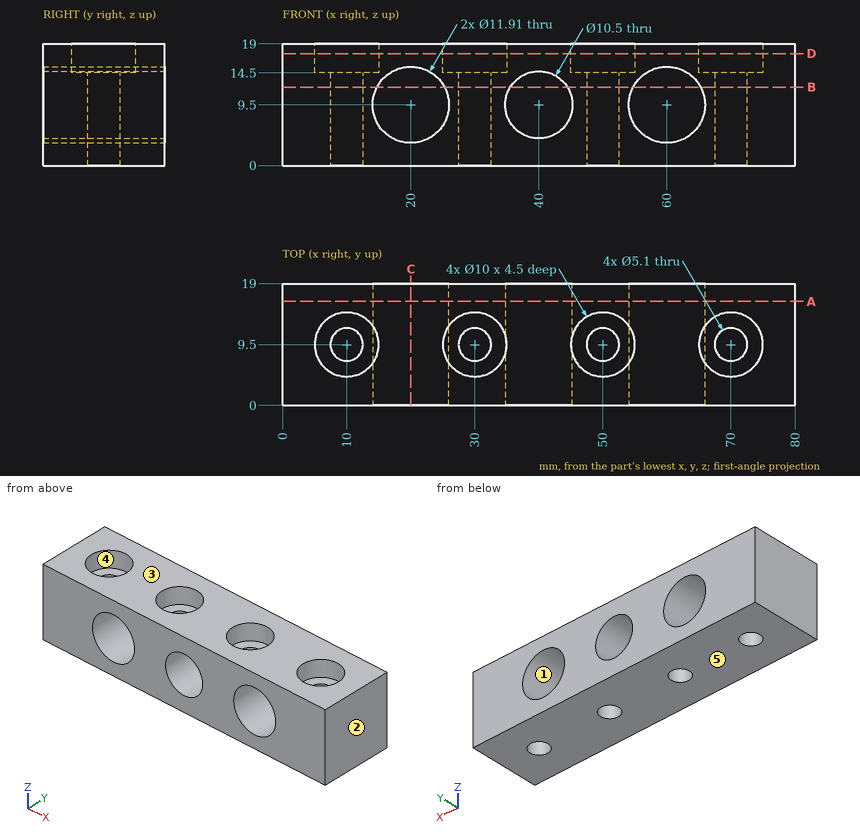
Answer from the drawing. Dimensions are ordinates in mm from the lowest x, y and z of the part. A direction names the side the tool comes from. Give positions to 0.01 mm unless a question says otherwise; leave off trailing zeros. Write each loop counter-clockwise with the first axis right and the second up, starting at its lowest first coordinate (ties: lowest second). Pieces come first, ordered by that corner, then holes. Notation, with made-up numbers: (-24, -15.5) - (9, -15.5) arc R20 ccw to (9, -8.5) - close; hole circle Ø8 at (-14, -36.5). An arc over 180 degrees is marked (long way). One line per item, written item: value. Start each with the question number.
1. Find section A-A (y = 16.25). Write down the section's boundary in (x, z) (3 decimals).
2. For the marked faces 4 and 5, determine the directions among +Z, -Z, +X, -X, +Y, -Y from which every point of the face is accessible in a straight line to the end or side of a thin tool.
3. For a pull along Z with two mould halves and no side action, classify the marked faces 1, 2 and 3 as +Z half, -Z half, draft (parallel to the pull), parting line (faces both ways), or undercut.
4. Find section B-B (z = 12.25). Write down the section's boundary in (x, y), then the cut area to 3 significant figures.
5. Consider probe 1 along X at (y, z) = (17.75, 9.75); probe 2 along Z at (x, y) = (60, 4) (3 decimals); probe 3 along X at (y, z) = (15.75, 6.5). Determine where each line is inside the solid, lowest interval first.
6. Find section C-C (x = 20). Write down the section's boundary in (y, z) (3 decimals), then the cut area to 3 significant figures.
7. Given pin 1 (8 mm diameter, centred on x = 30, y = 9.5, fed in from +Z); pin 2 (7 mm diameter, centred on x = 20, z = 9.5, fed in from +Y), each flat-ended and moving along its own axis, determine where each tip first touches the part or whether it passes through.
8. Find section D-D (z = 17.5). Write down the section's boundary in (x, y).
Geometry results:
1. outline: (0, 0) - (80, 0) - (80, 19) - (0, 19) - close; hole circle Ø11.91 at (20, 9.5); hole circle Ø10.5 at (40, 9.5); hole circle Ø11.91 at (60, 9.5)
2. face 4: +Z
2. face 5: -Z, +X, -X, +Y, -Y
3. face 1: undercut
3. face 2: draft
3. face 3: +Z half
4. outline: (0, 0) - (14.72, 0) - (14.72, 19) - (0, 19) - close; (25.28, 0) - (35.53, 0) - (35.53, 19) - (25.28, 19) - close; (44.47, 0) - (54.72, 0) - (54.72, 19) - (44.47, 19) - close; (65.28, 0) - (80, 0) - (80, 19) - (65.28, 19) - close; hole circle Ø5.1 at (10, 9.5); hole circle Ø5.1 at (30, 9.5); hole circle Ø5.1 at (50, 9.5); hole circle Ø5.1 at (70, 9.5)
4. area: 867 mm2
5. probe 1: 0 to 14.05, 25.95 to 34.76, 45.24 to 54.05, 65.95 to 80
5. probe 2: 0 to 3.545, 15.455 to 19
5. probe 3: 0 to 14.86, 25.14 to 35.69, 44.31 to 54.86, 65.14 to 80
6. outline: (0, 0) - (19, 0) - (19, 3.545) - (0, 3.545) - close; (0, 15.455) - (19, 15.455) - (19, 19) - (0, 19) - close
6. area: 135 mm2
7. pin 1: z = 14.5
7. pin 2: through
8. outline: (0, 0) - (80, 0) - (80, 19) - (0, 19) - close; hole circle Ø10 at (10, 9.5); hole circle Ø10 at (30, 9.5); hole circle Ø10 at (50, 9.5); hole circle Ø10 at (70, 9.5)
